from build123d import *

# Parameters (mm, degrees)
F1_DEPTH = 1.4
F2_W     = 1.3
F2_H     = 31
F2_H_2   = 24
F2_W_2   = 59
F2_H_3   = 1.4
F3_DEPTH = 1.75
F4_W     = 2.4
F4_H     = 31
F4_H_2   = 24
F4_W_2   = 59
F4_H_3   = 1.4
F5_DEPTH = 0.6


with BuildPart() as f1:
    # F0 (on Top) → F1 (new body)
    with BuildSketch(Plane.XY):
        Polygon((68.36, 0), (0, 0), (0, -24), (17.36, -24), (17.36, -27.5), (18.36, -31), (68.36, -31), align=None)
    extrude(amount=F1_DEPTH)

    # F2 (on face) → F3 (join)
    with BuildSketch(Plane(origin=(0, 0, 0), x_dir=(1, 0, 0), z_dir=(0, 0, -1))):
        with Locations((67.71, 15.5)):
            Rectangle(F2_W, F2_H)
        with Locations((0.65, 12)):
            Rectangle(F2_W, F2_H_2)
        with Locations((34.36, 0.7)):
            Rectangle(F2_W_2, F2_H_3)
    extrude(amount=F3_DEPTH)

    # F4 (on face) → F5 (join)
    with BuildSketch(Plane(origin=(0, 0, -1.75), x_dir=(1, 0, 0), z_dir=(0, 0, -1))):
        with Locations((67.16, 15.5)):
            Rectangle(F4_W, F4_H)
        with Locations((1.2, 12)):
            Rectangle(F4_W, F4_H_2)
        with Locations((34.36, 0.7)):
            Rectangle(F4_W_2, F4_H_3)
    extrude(amount=F5_DEPTH)


solid = f1.part
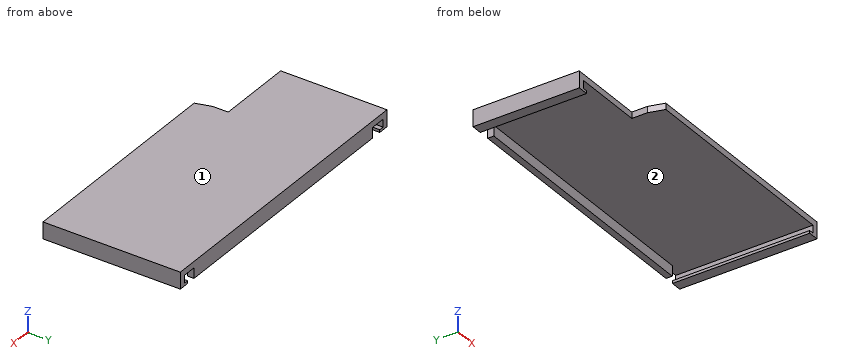
For this review, take the finished solid that the model builds, in its own axes (mm). Face numbers are marked on the shaded views. Round coordinates to 2 decimals unless told otherwise and drop trailing zeros. Order: outer loops, then holes, each group sorted by start corner. A loop starts at its lowest first (then second) coordinate and runs counter-clockwise, first axis right, second up. Notation, with made-up numbers: (6, 68) -> (57, 68) arc R32 cw to (57, 103) -> close; hole circle Ø4 at (41, -25.5). An arc over 180 degrees is marked (long way). Put each result on its own line as item: value.
Q1. Add section A-A on z = -1. Write out the cut boundary in (x, y).
Check result:
outline: (0, -24) -> (1.3, -24) -> (1.3, 0) -> (0, 0) -> close; (4.86, -1.4) -> (63.86, -1.4) -> (63.86, 0) -> (4.86, 0) -> close; (67.06, -31) -> (68.36, -31) -> (68.36, 0) -> (67.06, 0) -> close
Q2. Add section D-D on y = -25.5. Write out the cut boundary in (x, z).
Check result:
outline: (17.36, 0) -> (67.06, 0) -> (67.06, -1.75) -> (65.96, -1.75) -> (65.96, -2.35) -> (68.36, -2.35) -> (68.36, 1.4) -> (17.36, 1.4) -> close
Q3. Add section C-C on y = -7.5. Write out the cut boundary in (x, z).
Check result:
outline: (0, -2.35) -> (2.4, -2.35) -> (2.4, -1.75) -> (1.3, -1.75) -> (1.3, 0) -> (67.06, 0) -> (67.06, -1.75) -> (65.96, -1.75) -> (65.96, -2.35) -> (68.36, -2.35) -> (68.36, 1.4) -> (0, 1.4) -> close
Q4. Insertion check: pin 1 Ø1 at (x, y) = (33.5, -12.5) entering from -Z; pin 2 Ø1.9 at (x, z) = (32, -1.5) entering from -Y; pin 3 Ø1.1 at (y, z) = (-25.5, 0.5) entering from -X. Each pin has a flat end and moves straight along its axis. Give the tip position at first contact, or say it passes through.
Check result:
pin 1: z = 0
pin 2: y = -1.4
pin 3: x = 17.36
Q5. Mouldability with a two-part tool opening along X and no side actions: class the marked faces 1 and 2 as pulls with the +X half, pulls with the -X half, needs draft (parallel to the pull), parting line crosses it, or undercut.
Check result:
face 1: needs draft
face 2: undercut
Q6. For probe 1 along X at (y, z) = (-22.5, -0.6); probe 2 along Y at (x, z) = (53.5, -1.3); probe 3 along X at (y, z) = (-23.5, -1.95), list the stretches that pass through material, from the lowest coordinate up. Write a range as [from, to].
Check result:
probe 1: [0, 1.3], [67.06, 68.36]
probe 2: [-1.4, 0]
probe 3: [0, 2.4], [65.96, 68.36]
Q7. Add section B-B on x = 45.5. Write out the cut boundary in (y, z).
Check result:
outline: (-31, 0) -> (-1.4, 0) -> (-1.4, -2.35) -> (0, -2.35) -> (0, 1.4) -> (-31, 1.4) -> close
